For this review, take the finished solid that the model builds, in its own axes (mm). A direction names the side the tool comes from. Coordinates: 2 decimals unless noted, no trailing zeros. Write each loop counter-clockwise with the first axis right and the second up, starting at its lowest first coordinate (ties: lowest second). Pieces come first, ordered by that corner, then holes.
```python
from build123d import *

# Parameters (mm, degrees)
BOSS_EXTRUDE1_DEPTH      = 3.175
BOSS_EXTRUDE1_DEPTH_BACK = 3.175
SKETCH1_R                = 6.35


with BuildPart() as part:
    # Sketch1 → Boss-Extrude1 (new, two sides: drawn at the far end of the back side and taken through both)
    with BuildSketch(Plane.XY.offset(-BOSS_EXTRUDE1_DEPTH_BACK)):
        with BuildLine():
            ThreePointArc((5.798103615, 18.146197797), (3.716470634, 18.683959592), (1.5875, 18.98373893))
            Line((1.5875, 18.98373893), (1.5875, 12.7))
            Line((1.5875, 12.7), (-1.5875, 12.7))
            Line((-1.5875, 12.7), (-1.5875, 18.98373893))
            ThreePointArc((-1.5875, 18.98373893), (-3.716470634, 18.683959592), (-5.798103615, 18.146197797))
            Line((-5.798103615, 18.146197797), (-3.393420833, 12.340780012))
            Line((-3.393420833, 12.340780012), (-6.326738349, 11.125760114))
            Line((-6.326738349, 11.125760114), (-8.731421131, 16.931177899))
            ThreePointArc((-8.731421131, 16.931177899), (-10.583612939, 15.839496114), (-12.300998514, 14.546062545))
            Line((-12.300998514, 14.546062545), (-7.857724106, 10.102788136))
            Line((-7.857724106, 10.102788136), (-10.102788136, 7.857724106))
            Line((-10.102788136, 7.857724106), (-14.546062545, 12.300998514))
            ThreePointArc((-14.546062545, 12.300998514), (-15.839496114, 10.583612939), (-16.931177899, 8.731421131))
            Line((-16.931177899, 8.731421131), (-11.125760114, 6.326738349))
            Line((-11.125760114, 6.326738349), (-12.340780012, 3.393420833))
            Line((-12.340780012, 3.393420833), (-18.146197797, 5.798103615))
            ThreePointArc((-18.146197797, 5.798103615), (-18.683959592, 3.716470634), (-18.98373893, 1.5875))
            Line((-18.98373893, 1.5875), (-12.7, 1.5875))
            Line((-12.7, 1.5875), (-12.7, -1.5875))
            Line((-12.7, -1.5875), (-18.98373893, -1.5875))
            ThreePointArc((-18.98373893, -1.5875), (-18.683959592, -3.716470634), (-18.146197797, -5.798103615))
            Line((-18.146197797, -5.798103615), (-12.340780012, -3.393420833))
            Line((-12.340780012, -3.393420833), (-11.125760114, -6.326738349))
            Line((-11.125760114, -6.326738349), (-16.931177899, -8.731421131))
            ThreePointArc((-16.931177899, -8.731421131), (-15.839496114, -10.583612939), (-14.546062545, -12.300998514))
            Line((-14.546062545, -12.300998514), (-10.102788136, -7.857724106))
            Line((-10.102788136, -7.857724106), (-7.857724106, -10.102788136))
            Line((-7.857724106, -10.102788136), (-12.300998514, -14.546062545))
            ThreePointArc((-12.300998514, -14.546062545), (-10.583612939, -15.839496114), (-8.731421131, -16.931177899))
            Line((-8.731421131, -16.931177899), (-6.326738349, -11.125760114))
            Line((-6.326738349, -11.125760114), (-3.393420833, -12.340780012))
            Line((-3.393420833, -12.340780012), (-5.798103615, -18.146197797))
            ThreePointArc((-5.798103615, -18.146197797), (-3.716470634, -18.683959592), (-1.5875, -18.98373893))
            Line((-1.5875, -18.98373893), (-1.5875, -12.7))
            Line((-1.5875, -12.7), (1.5875, -12.7))
            Line((1.5875, -12.7), (1.5875, -18.98373893))
            ThreePointArc((1.5875, -18.98373893), (3.716470634, -18.683959592), (5.798103615, -18.146197797))
            Line((5.798103615, -18.146197797), (3.393420833, -12.340780012))
            Line((3.393420833, -12.340780012), (6.326738349, -11.125760114))
            Line((6.326738349, -11.125760114), (8.731421131, -16.931177899))
            ThreePointArc((8.731421131, -16.931177899), (10.583612939, -15.839496114), (12.300998514, -14.546062545))
            Line((12.300998514, -14.546062545), (7.857724106, -10.102788136))
            Line((7.857724106, -10.102788136), (10.102788136, -7.857724106))
            Line((10.102788136, -7.857724106), (14.546062545, -12.300998514))
            ThreePointArc((14.546062545, -12.300998514), (15.839496114, -10.583612939), (16.931177899, -8.731421131))
            Line((16.931177899, -8.731421131), (11.125760114, -6.326738349))
            Line((11.125760114, -6.326738349), (12.340780012, -3.393420833))
            Line((12.340780012, -3.393420833), (18.146197797, -5.798103615))
            ThreePointArc((18.146197797, -5.798103615), (18.683959592, -3.716470634), (18.98373893, -1.5875))
            Line((18.98373893, -1.5875), (12.7, -1.5875))
            Line((12.7, -1.5875), (12.7, 1.5875))
            Line((12.7, 1.5875), (18.98373893, 1.5875))
            ThreePointArc((18.98373893, 1.5875), (18.683959592, 3.716470634), (18.146197797, 5.798103615))
            Line((18.146197797, 5.798103615), (12.340780012, 3.393420833))
            Line((12.340780012, 3.393420833), (11.125760114, 6.326738349))
            Line((11.125760114, 6.326738349), (16.931177899, 8.731421131))
            ThreePointArc((16.931177899, 8.731421131), (15.839496114, 10.583612939), (14.546062545, 12.300998514))
            Line((14.546062545, 12.300998514), (10.102788136, 7.857724106))
            Line((10.102788136, 7.857724106), (7.857724106, 10.102788136))
            Line((7.857724106, 10.102788136), (12.300998514, 14.546062545))
            ThreePointArc((12.300998514, 14.546062545), (10.583612939, 15.839496114), (8.731421131, 16.931177899))
            Line((8.731421131, 16.931177899), (6.326738349, 11.125760114))
            Line((6.326738349, 11.125760114), (3.393420833, 12.340780012))
            Line((3.393420833, 12.340780012), (5.798103615, 18.146197797))
        make_face()
        Circle(SKETCH1_R, mode=Mode.SUBTRACT)
    extrude(amount=BOSS_EXTRUDE1_DEPTH + BOSS_EXTRUDE1_DEPTH_BACK)


solid = part.part
```
1) Consider section C-C (y = 13.5). Give the boundary of the cut face in (x, z) (1 decimal), then the cut area to 3 significant figures.
2) For L1, parallel to Y at x = 0, z = -2; L2, parallel to X at y = 15, z = 1; L3, parallel to Y at x = -9.5, z = 2.5, list the stretches that pass through material, from the lowest coordinate up.
3) Consider section D-D (y = 7). Give the boundary of the cut face in (x, z) (3 decimals).
4) Tool access review of faces 4 (the face through (-14.069, 7.546, -0.044)), 5 (the face through (-4.61, 15.28, -0.04)), 6 (the face through (-1.588, -16, 0)): name each direction out of +Z, -Z, +X, -X, +Y, -Y from which nothing blocks a thin tool from reaching the whole face with its end or side.
5) The part is to be moulded in two halves that separate along X. For faces 1 (the face through (-13.988, -7.512, -0.044)), 2 (the face through (-9, -8.96, -0.04)), 3 (the face through (16, -1.588, 0)), say which applies: pulls with the +X half, pulls with the -X half, needs draft (parallel to the pull), parting line crosses it, or undercut.
6) Consider section A-A (x = 0). Give the boundary of the cut face in (y, z) (3 decimals).
7) Clearance check with flat-ended pins moving along their axes: P1, Ø1.6, axis at y = -0.5, z = 1.5, coming from the -X side; P2, Ø1.5, axis at x = -10.5, z = 0, coming from the +Y side; P3, Ø1.9, axis at y = 14.5, z = 1, coming from the -X side. State where each tip first meets the part, or that it passes through.
Results:
1. outline: (-11.3, -3.2) - (-7.3, -3.2) - (-7.3, 3.2) - (-11.3, 3.2) - close; (-3.9, -3.2) - (-1.6, -3.2) - (-1.6, 3.2) - (-3.9, 3.2) - close; (1.6, -3.2) - (3.9, -3.2) - (3.9, 3.2) - (1.6, 3.2) - close; (7.3, -3.2) - (11.3, -3.2) - (11.3, 3.2) - (7.3, 3.2) - close
1. area: 79.1 mm2
2. L1: y = -12.7 to -6.35, 6.35 to 12.7
2. L2: x = -11.74 to -7.93, -4.49 to -1.59, 1.59 to 4.49, 7.93 to 11.74
2. L3: y = -16.51 to -11.75, -8.46 to 8.46, 11.75 to 16.51
3. outline: (-12.751, -3.175) - (12.751, -3.175) - (12.751, 3.175) - (-12.751, 3.175) - close
4. face 4: +Z, -Z, -X
4. face 5: +Z, -Z
4. face 6: +Z, -Z, -Y
5. face 1: pulls with the -X half
5. face 2: undercut
5. face 3: needs draft
6. outline: (-12.7, -3.175) - (-6.35, -3.175) - (-6.35, 3.175) - (-12.7, 3.175) - close; (6.35, -3.175) - (12.7, -3.175) - (12.7, 3.175) - (6.35, 3.175) - close
7. P1: stops at x = -12.7
7. P2: stops at y = 16.37
7. P3: stops at x = -12.3
